Geometry check sheet. Reference: drawing and pictorial views, mm from the part's lowest x, y, z. Give positions to 0.01 mm unless a question says otherwise; leave off trailing zeros. Loops run counter-clockwise (first coordinate to the right, second up) from the corner with the lowest first, then second, coordinate; pieces in that order, holes last. Notation, with made-up numbers: (-39, 15.5) - (-12, 15.5) arc R25 cw to (-12, 45.5) - close; hole circle Ø6 at (64, 36.5). An arc over 180 degrees is marked (long way). Answer in a Markdown table with one row per item. Add a question column.
(1) Go/stop test with a flat-tipped pin: P1, Ø8.5, axis at x = 20.81, y = 32.53, coming from the +Z side. Record where the tip stops, or that it passes through.
(2) Sectioned sample at C-C on x = 167.5. Enter the section's corners in (y, z).
(3) Sectioned sample at B-B on y = 106. Enter the section's corners in (x, z).
(4) Thickness scan on L1, parallel to Y at x = 109.5, z = 1.8 (1 decimal); L2, parallel to X at y = 114, z = 0.3 (1 decimal); L3, parallel to X at y = 81, z = 2. Record the ranges inside material, lowest first.
(5) Sectioned sample at A-A on z = 2.05. Enter the section's corners in (x, y), then the cut area to 3 significant figures.
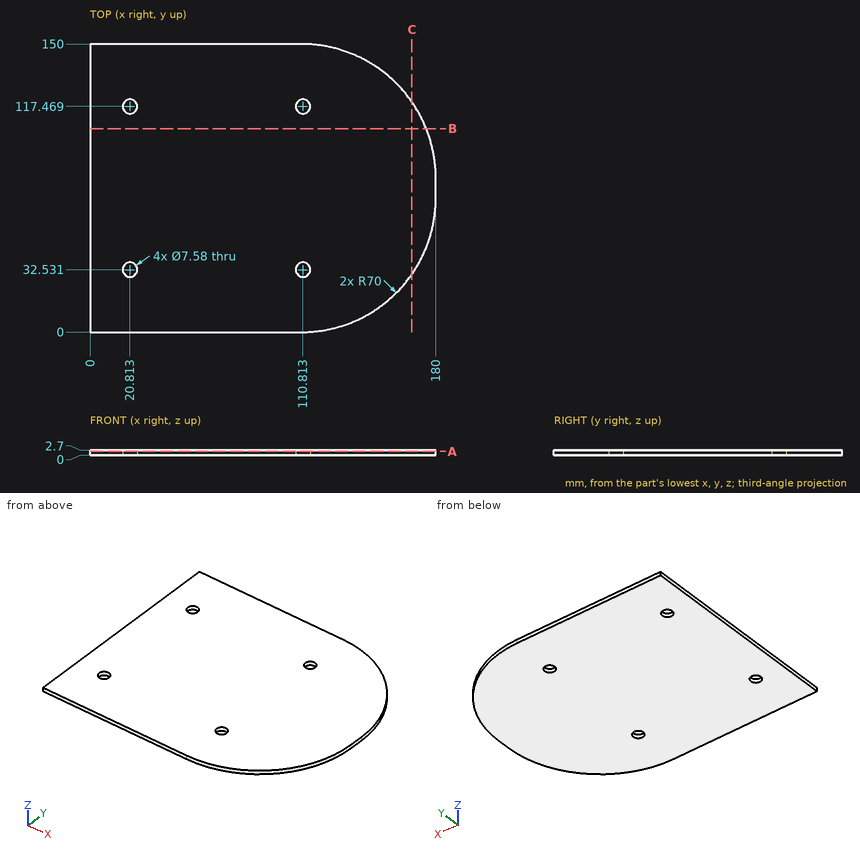
Reply:
| question | item | result |
|---|---|---|
| 1 | P1 | z = 2.7 |
| 2 | outline | (30.08, 0) - (119.92, 0) - (119.92, 2.7) - (30.08, 2.7) - close |
| 3 | outline | (0, 0) - (174.99, 0) - (174.99, 2.7) - (0, 2.7) - close |
| 4 | L1 | 0 to 29, 36.1 to 113.9, 121 to 150 |
| 4 | L2 | 0 to 19.3, 22.3 to 109.3, 112.3 to 171.2 |
| 4 | L3 | 0 to 179.99 |
| 5 | outline | (0, 0) - (110, 0) arc R70 ccw to (180, 70) - (180, 80) arc R70 ccw to (110, 150) - (0, 150) - close; hole circle Ø7.58 at (20.81, 32.53); hole circle Ø7.58 at (20.81, 117.47); hole circle Ø7.58 at (110.81, 32.53); hole circle Ø7.58 at (110.81, 117.47) |
| 5 | area | 24,700 mm^2 |
